Can you work these out from the model? Positions are in its coordinate system, mm. Face numbers are marked on the shaded views. A direction names the side the tool comes from. Round coordinates to 2 decimals unless told otherwise and drop trailing zeros. Write each loop counter-clockwise with the first axis right and the second up, starting at its lowest first coordinate (ties: lowest second). Pieces come first, ordered by that corner, then holes. Notation, with made-up numbers: (38, 19) - (87, 19) arc R13 ccw to (87, 23) - close; hole circle Ø9 at (12, 35.5). An arc over 180 degrees is marked (long way). One line per item, written item: value. Start each with the question number.
(1) I want a section at C-C on z = -0.6. List the corners of the cut face in (x, y) for me.
(2) I'm going to push flat-ended pins straight in: pin 1 Ø3 at (x, y) = (1.5, -6) entering from -Z; pin 2 Ø4 at (x, y) = (-2.5, -8) entering from -Z; pin 3 Ø1 at (y, z) = (-10.5, -0.5) entering from +X. Where does each tip first touch, or does it pass through?
(3) I want a section at A-A on x = 0. List the corners of the cut face in (y, z) for me, plus the area to 3 significant figures.
(4) I want a section at B-B on y = -0.25. List the corners of the cut face in (x, z) for me.
(5) If I drill on L1, parallel to X at y = 0, z = -0.45; L2, parallel to X at y = -11.5, z = 0.05; L3, parallel to X at y = 1, z = -0.35, over which ranges is the centre line in solid material (lowest first)? Write a range as from..to.
(6) On a 3-axis mill with a long thin cutter (end or side, diameter ignored), from which of +Z, -Z, +X, -X, +Y, -Y can I reach the whole of each face in a straight line? I mean the marked faces 5, 6 and 7. Say none if no direction works.
(7) Thinking about a two-plate mould opening in Y: for the marked faces 1, 2, 3 and 4, which applies, +Y half, -Y half, draft (parallel to the pull), parting line (faces both ways), or undercut?
(8) I want a section at D-D on x = 3.75. List the corners of the cut face in (y, z) for me, plus the area to 3 significant figures.
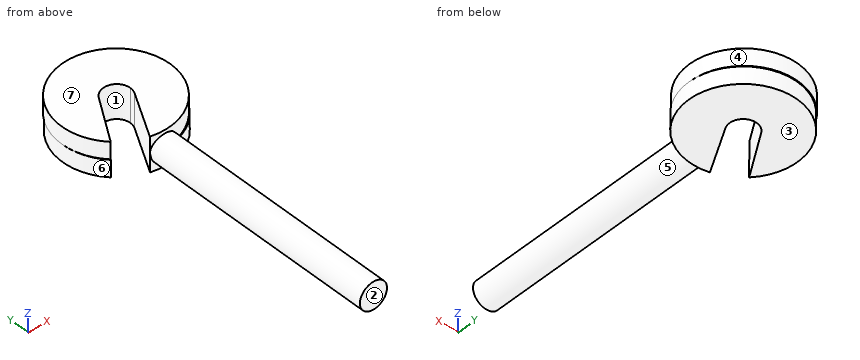
from build123d import *

# Parameters (mm, degrees)
F0_R     = 1
F1_DEPTH = 19.05
F2_R     = 4
F3_DEPTH = 1.25
F4_R     = 4
F5_DEPTH = 1.25
F7_DEPTH = 25
F8_DEPTH = 25


with BuildPart() as f1:
    # F0 (on Front) → F1 (new body)
    with BuildSketch(Plane.XZ):
        Circle(F0_R)
    extrude(amount=F1_DEPTH)

    # F2 (on Top) → F3 (join)
    with BuildSketch(Plane.XY):
        with Locations((0, 2)):
            Circle(F2_R)
    extrude(amount=F3_DEPTH)

    # F4 (on Top) → F5 (join)
    with BuildSketch(Plane.XY):
        with Locations((0, 1.933241)):
            Circle(F4_R)
    extrude(amount=-F5_DEPTH)

    # F6 (on face) → F7 (cut)
    with BuildSketch(Plane(origin=(0, 0, -1.25), x_dir=(1, 0, 0), z_dir=(0, 0, -1))):
        with BuildLine():
            ThreePointArc((-0.845681, -2.46693), (0.277776, -2.893887), (1, -1.933241))
            ThreePointArc((1, -1.933241), (0.967302, -1.679612), (0.871344, -1.442569))
            Line((0.871344, -1.442569), (-0.845681, -2.46693))
        make_face()
        with BuildLine():
            Line((-0.845681, -2.46693), (0.871344, -1.442569))
            ThreePointArc((0.871344, -1.442569), (-0.512341, -1.074459), (-0.845681, -2.46693))
        make_face()
    extrude(amount=-F7_DEPTH, mode=Mode.SUBTRACT)

    # F6 (on face) → F8 (cut)
    with BuildSketch(Plane(origin=(0, 0, -1.25), x_dir=(1, 0, 0), z_dir=(0, 0, -1))):
        with BuildLine():
            ThreePointArc((-0.845681, -2.46693), (-0.512341, -1.074459), (0.871344, -1.442569))
            Line((0.871344, -1.442569), (-1.029019, 1.932134))
            ThreePointArc((-1.029019, 1.932134), (-2.049337, 1.501904), (-2.912605, 0.808425))
            Line((-2.912605, 0.808425), (-0.845681, -2.46693))
        make_face()
    extrude(amount=-F8_DEPTH, mode=Mode.SUBTRACT)


solid = f1.part
Established:
1. outline: (-2.91, -0.81) - (-0.85, 2.47) arc R1 cw to (1, 1.93) arc R1 cw to (0.87, 1.44) - (-1.03, -1.93) arc R4 ccw to (-0.8, -1.99) - (-0.8, -19.05) - (0.8, -19.05) - (0.8, -1.99) arc R4 ccw (long way) to start
2. pin 1: z = -1
2. pin 2: z = -0.87
2. pin 3: x = 1
3. outline: (-19.05, -1) - (-2.07, -1) - (-2.07, -1.25) - (-0.1, -1.25) - (-0.1, 1.25) - (-2, 1.25) - (-2, 1) - (-19.05, 1) - close; (2.93, -1.25) - (5.93, -1.25) - (5.93, 0) - (6, 0) - (6, 1.25) - (2.93, 1.25) - close
3. area: 46.4 mm2
4. outline: (-3.35, -1.25) - (-2.56, -1.25) - (-2.56, 1.25) - (-3.31, 1.25) - (-3.31, 0) - (-3.35, 0) - close; (-0.08, -1.25) - (3.35, -1.25) - (3.35, 0) - (3.31, 0) - (3.31, 1.25) - (-0.08, 1.25) - close
5. L1: -3.5..-2.4, 0.06..3.5
5. L2: -1..1
5. L3: -3.89..-1.77, 0.62..3.89
6. face 5: -Y
6. face 6: -Z
6. face 7: +Z, +X, -X, +Y, -Y
7. face 1: undercut
7. face 2: -Y half
7. face 3: draft
7. face 4: parting line
8. outline: (0.54, -1.25) - (3.33, -1.25) - (3.33, 0) - (3.39, 0) - (3.39, 1.25) - (0.61, 1.25) - (0.61, 0) - (0.54, 0) - close
8. area: 6.96 mm2
